from build123d import *

# Parameters (mm, degrees)
ESQUISSE1_R        = 44
BOSS_EXTRU_1_DEPTH = 160
ESQUISSE2_R        = 15
BOSS_EXTRU_2_DEPTH = 50
ESQUISSE3_R        = 17.5
BOSS_EXTRU_3_DEPTH = 6
CONG_1_R           = 14
CONG_2_R           = 14
CONG_3_R           = 14


with BuildPart() as part:
    # Esquisse1 → Boss.-Extru.1 (new body)
    with BuildSketch(Plane(origin=(0, 0, 0), x_dir=(1, 0, 0), z_dir=(0, 1, 0))):
        with Locations(Location((0, 0, 0), (0, 0, 270))):
            Circle(ESQUISSE1_R)
    extrude(amount=BOSS_EXTRU_1_DEPTH)

    # Esquisse2 → Boss.-Extru.2 (add)
    with BuildSketch(Plane(origin=(0, 160, 0), x_dir=(1, 0, 0), z_dir=(0, 1, 0))):
        with Locations(Location((0, 0, 0), (0, 0, 270))):
            Circle(ESQUISSE2_R)
    extrude(amount=BOSS_EXTRU_2_DEPTH)

    # Esquisse3 → Boss.-Extru.3 (add)
    with BuildSketch(Plane(origin=(0, 210, 0), x_dir=(1, 0, 0), z_dir=(0, 1, 0))):
        with Locations(Location((0, 0, 0), (0, 0, 270))):
            Circle(ESQUISSE3_R)
    extrude(amount=BOSS_EXTRU_3_DEPTH)

    # Congé1
    cong_1_edges = [part.edges().sort_by_distance(p)[0] for p in [
        (0, 160, -44),
        (0, 160, -15),
    ]]
    fillet(cong_1_edges, radius=CONG_1_R)

    # Congé2
    # the kernel refuses this fillet: 14 mm, written as the material it adds along each edge
    with BuildSketch(Plane(origin=(0, 210, 0), x_dir=(0, 0, 1), z_dir=(-1, 0, 0))) as cong_2_piece_1:
        with BuildLine():
            CenterArc((29, -7.984359711), CONG_2_R, 145.228055968, 34.771944032)
            Line((17.5, 0), (17.27, 0.159687194))
            ThreePointArc((17.27, 0.159687194), (16.25, 0.28), (15, 0.28))
            Line((15, 0.28), (14.72, 0))
            Line((14.72, 0), (14.72, -7.984359711))
            Line((14.72, -7.984359711), (15, -7.984359711))
        make_face()
    revolve(axis=Axis((0, 210, 0), (0, 1, 0)))

    # Congé3
    cong_3_edges = [part.edges().sort_by_distance(p)[0] for p in [
        (0, 0, -44),
    ]]
    fillet(cong_3_edges, radius=CONG_3_R)


solid = part.part
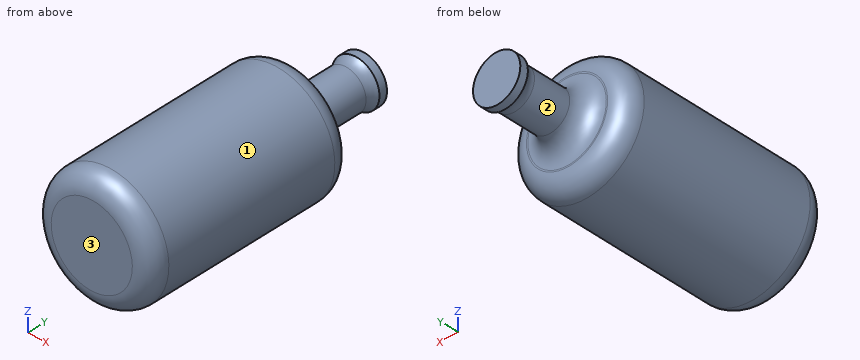
Work out the finished part from the listing and answer in its coordinate system (mm). Face numbers are marked on the shaded views. Round coordinates to 2 decimals unless told otherwise and drop trailing zeros. Loops run counter-clockwise (first coordinate to the right, second up) from the corner with the lowest first, then second, coordinate; pieces in that order, holes last. Notation, with made-up numbers: M -31,-27 L -14,-27 A21 cw -14,-20 Z; hole C -19,47 d8. An arc over 180 degrees is marked long. One line per question, with ' | ' between items. Start each with the question number.
(1) For a pull along Y with two mould halves and no side action, classify the marked faces 1, 2 and 3 as released by +Y, released by -Y, zero draft, split by the parting line, or undercut.
(2) Flat-ended cylindrical pins translate along their axes: pin 1 Ø12 at (x, z) = (22.5, -19) entering from +Y; pin 2 Ø8 at (x, y) = (6.5, 67) entering from +Z; pin 3 Ø6 at (x, z) = (-29, -21) entering from +Y. Find the tip coordinate at first contact, or state that the pin passes through.
(3) A cutting plane is placed at A-A on x = 0. Write down the section's boundary in (y, z).
(4) A cutting plane is placed at C-C on y = 189. Write down the section's boundary in (x, z).
(5) Find the intervals of material crossed by line 1 (Y direction, x = 7.5, z = -29); line 2 (Z direction, x = 34.5, y = 22); line 3 (X direction, y = 72.5, z = 9), in increasing order.
(6) A cutting plane is placed at B-B on z = 0. Write down the section's boundary in (x, y), plus the area to 3 significant figures.
(7) A cutting plane is placed at D-D on y = 18. Write down the section's boundary in (x, z), plus the area to 3 significant figures.
Geometry check:
1) face 1: zero draft | face 2: undercut | face 3: released by -Y
2) pin 1: stops at y = 161.15 | pin 2: stops at z = 43.93 | pin 3: stops at y = 159.72
3) outline: M 0,-30 A14 ccw 14,-44 L 146,-44 A14 ccw 160,-30 L 160,-29 A14 cw 174,-15 L 202.02,-15 A14 cw 210,-17.5 L 216,-17.5 L 216,17.5 L 210,17.5 A14 cw 202.02,15 L 174,15 A14 cw 160,29 L 160,30 A14 ccw 146,44 L 14,44 A14 ccw 0,30 Z
4) outline: C 0,0 d30
5) line 1: y = 0 to 160 | line 2: z = -27.31 to 27.31 | line 3: x = -43.07 to 43.07
6) outline: M -44,14 A14 ccw -30,0 L 30,0 A14 ccw 44,14 L 44,146 A14 ccw 30,160 L 29,160 A14 cw 15,174 L 15,202.02 A14 cw 17.5,210 L 17.5,216 L -17.5,216 L -17.5,210 A14 cw -15,202.02 L -15,174 A14 cw -29,160 L -30,160 A14 ccw -44,146 Z | area: 15,700 mm²
7) outline: C 0,0 d88 | area: 6,080 mm²
